Could you check a few things on this model? Use its own coordinates, in mm. Face numbers are marked on the shaded views. A direction names the side the tool comes from. Give positions to 0.01 mm unless a question says otherwise; leave off trailing zeros. Loops run counter-clockwise (first coordinate to the right, second up) from the corner with the lowest first, then second, coordinate; pieces in that order, holes last. Notation, with made-up numbers: M 73.5,-12 L 78.5,-12 A15 cw 78.5,8 Z; hole C -6,-14.75 d7. An arc over 180 degrees is marked long. Answer in a Markdown table with one row per item. Add a question column.
```python
from build123d import *

# Parameters (mm, degrees)
F0_R     = 3
F1_DEPTH = 18.2
F3_DEPTH = 8.5
F5_DEPTH = 14.6
F6_R     = 0.5
F7_DEPTH = 0.5


with BuildPart() as f1:
    # F0 (on Front) → F1 (new body)
    with BuildSketch(Plane.XZ):
        with BuildLine():
            Line((-15.090977, -27.410671), (-15.090977, -30.910671))
            Line((-15.090977, -30.910671), (-3.590977, -30.910671))
            Line((-3.590977, -30.910671), (-3.590977, -27.410671))
            Line((-3.590977, -27.410671), (-2.840977, -27.410671))
            Line((-2.840977, -27.410671), (-2.840977, -24.910671))
            Line((-2.840977, -24.910671), (-3.590977, -24.910671))
            Line((-3.590977, -24.910671), (-4.440977, -24.910671))
            ThreePointArc((-4.440977, -24.910671), (-5.699463, -22.199699), (-8.290977, -20.710671))
            Line((-8.290977, -20.710671), (-8.290977, -21.210671))
            Line((-8.290977, -21.210671), (-10.390977, -21.210671))
            Line((-10.390977, -21.210671), (-10.390977, -20.710671))
            ThreePointArc((-10.390977, -20.710671), (-12.982492, -22.199699), (-14.240977, -24.910671))
            Line((-14.240977, -24.910671), (-15.090977, -24.910671))
            Line((-15.090977, -24.910671), (-15.840977, -24.910671))
            Line((-15.840977, -24.910671), (-15.840977, -27.410671))
            Line((-15.840977, -27.410671), (-15.090977, -27.410671))
        make_face()
        with Locations((-9.340977, -25.910671)):
            Circle(F0_R, mode=Mode.SUBTRACT)
    extrude(amount=F1_DEPTH)

    # F2 (on face) → F3 (join)
    with BuildSketch(Plane.XZ.offset(18.2)):
        with BuildLine():
            Line((-15.090977, -27.410671), (-15.090977, -30.910671))
            Line((-15.090977, -30.910671), (-3.590977, -30.910671))
            Line((-3.590977, -30.910671), (-3.590977, -27.410671))
            Line((-3.590977, -27.410671), (-2.840977, -27.410671))
            Line((-2.840977, -27.410671), (-2.840977, -24.910671))
            Line((-2.840977, -24.910671), (-3.590977, -24.910671))
            Line((-3.590977, -24.910671), (-4.440977, -24.910671))
            ThreePointArc((-4.440977, -24.910671), (-5.699463, -22.199699), (-8.290977, -20.710671))
            Line((-8.290977, -20.710671), (-8.290977, -21.210671))
            Line((-8.290977, -21.210671), (-10.390977, -21.210671))
            Line((-10.390977, -21.210671), (-10.390977, -20.710671))
            ThreePointArc((-10.390977, -20.710671), (-12.982492, -22.199699), (-14.240977, -24.910671))
            Line((-14.240977, -24.910671), (-15.090977, -24.910671))
            Line((-15.090977, -24.910671), (-15.840977, -24.910671))
            Line((-15.840977, -24.910671), (-15.840977, -27.410671))
            Line((-15.840977, -27.410671), (-15.090977, -27.410671))
        make_face()
    extrude(amount=F3_DEPTH)

    # F4 (on face) → F5 (join)
    with BuildSketch(Plane.XZ.offset(26.7)):
        with BuildLine():
            Line((-15.090977, -27.410671), (-15.090977, -30.910671))
            Line((-15.090977, -30.910671), (-3.590977, -30.910671))
            Line((-3.590977, -30.910671), (-3.590977, -27.410671))
            Line((-3.590977, -27.410671), (-2.840977, -27.410671))
            Line((-2.840977, -27.410671), (-2.840977, -24.910671))
            Line((-2.840977, -24.910671), (-3.590977, -24.910671))
            Line((-3.590977, -24.910671), (-4.440977, -24.910671))
            ThreePointArc((-4.440977, -24.910671), (-5.699463, -22.199699), (-8.290977, -20.710671))
            Line((-8.290977, -20.710671), (-8.290977, -21.210671))
            Line((-8.290977, -21.210671), (-10.390977, -21.210671))
            Line((-10.390977, -21.210671), (-10.390977, -20.710671))
            ThreePointArc((-10.390977, -20.710671), (-12.982492, -22.199699), (-14.240977, -24.910671))
            Line((-14.240977, -24.910671), (-15.090977, -24.910671))
            Line((-15.090977, -24.910671), (-15.840977, -24.910671))
            Line((-15.840977, -24.910671), (-15.840977, -27.410671))
            Line((-15.840977, -27.410671), (-15.090977, -27.410671))
        make_face()
        with BuildLine():
            ThreePointArc((-11.577045, -27.910671), (-9.340977, -22.910671), (-7.104909, -27.910671))
            Line((-7.104909, -27.910671), (-5.340977, -27.910671))
            Line((-5.340977, -27.910671), (-5.340977, -28.910671))
            Line((-5.340977, -28.910671), (-8.840977, -28.910671))
            Line((-8.840977, -28.910671), (-8.840977, -30.310671))
            Line((-8.840977, -30.310671), (-9.840977, -30.310671))
            Line((-9.840977, -30.310671), (-9.840977, -28.910671))
            Line((-9.840977, -28.910671), (-13.340977, -28.910671))
            Line((-13.340977, -28.910671), (-13.340977, -27.910671))
            Line((-13.340977, -27.910671), (-11.577045, -27.910671))
        make_face(mode=Mode.SUBTRACT)
    extrude(amount=F5_DEPTH)

    # F6 (on face) → F7 (cut)
    with BuildSketch(Plane(origin=(0, 0, -30.910671), x_dir=(1, 0, 0), z_dir=(0, 0, -1))):
        with Locations((-13.090977, 39.3)):
            Circle(F6_R)
    extrude(amount=-F7_DEPTH, mode=Mode.SUBTRACT)


solid = f1.part
```
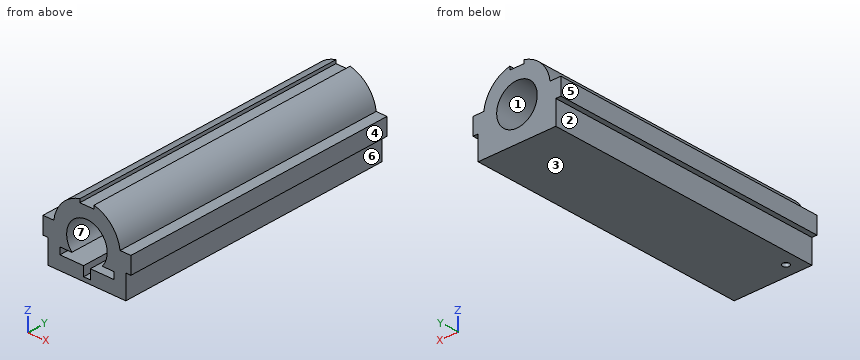
Item 1: Suppose I cut it at C-C (y = -39.3). List the corners of the cut face in (x, z) for me.
Item 2: For P1, Ø0.6, axis at x = -15.5, y = -15.5, coming from the -Z side; P2, Ø1, axis at y = -20, z = -28.5, coming from the -X side; P3, Ø0.6, axis at y = -27, z = -21, coming from the +X side, each with a flat end and sliding along its axis, tell me the tip position at first contact or that it passes through.
Item 3: I need wall thicknesses on L1, parallel to Z at x = -9.5, y = -13; L2, parallel to X at y = -31, z = -30; L3, parallel to Z at x = -9.25, y = -29. Which ranges of each line are inside material? Lowest first, please.
Item 4: For the marked faces 5, 6 and 7, which set-ups out of +Z, -Z, +X, -X, +Y, -Y let a thin tool reach every point of the face, with its end or its side?
Item 5: Suppose I cut it at B-B (z = -29.5). List the corners of the cut face in (x, y) for me, then the cut area to 3 significant figures.
Item 6: Suppose I cut it at A-A (y = -27.5). List the corners of the cut face in (x, z) for me, then the cut area to 3 significant figures.
Item 7: Suppose I cut it at D-D (y = -16). List the corners of the cut face in (x, z) for me.
Item 8: If we mould it in two halves opening along X, with no side actions, what happens to the marked faces 1, 2, 3 and 4? For each: +X half, -X half, draft (parallel to the pull), parting line (faces both ways), or undercut.
Values found:
| question | item | result |
|---|---|---|
| 1 | outline | M -15.84,-27.41 L -15.09,-27.41 L -15.09,-30.91 L -13.59,-30.91 L -13.59,-30.41 L -12.59,-30.41 L -12.59,-30.91 L -3.59,-30.91 L -3.59,-27.41 L -2.84,-27.41 L -2.84,-24.91 L -4.44,-24.91 A4.94 ccw -8.29,-20.71 L -8.29,-21.21 L -10.39,-21.21 L -10.39,-20.71 A4.94 ccw -14.24,-24.91 L -15.84,-24.91 Z; hole M -13.34,-28.91 L -9.84,-28.91 L -9.84,-30.31 L -8.84,-30.31 L -8.84,-28.91 L -5.34,-28.91 L -5.34,-27.91 L -7.1,-27.91 A3 ccw long -11.58,-27.91 L -13.34,-27.91 Z |
| 2 | P1 | z = -27.41 |
| 2 | P2 | x = -15.09 |
| 2 | P3 | x = -6.8 |
| 3 | L1 | -30.91 to -28.91, -22.91 to -21.21 |
| 3 | L2 | -15.09 to -9.84, -8.84 to -3.59 |
| 3 | L3 | -30.91 to -30.31, -22.91 to -21.21 |
| 4 | face 5 | +Z, -Z, -X, +Y, -Y |
| 4 | face 6 | -Z, +X, +Y, -Y |
| 4 | face 7 | -Y |
| 5 | outline | M -15.09,-41.3 L -9.84,-41.3 L -9.84,-26.7 L -8.84,-26.7 L -8.84,-41.3 L -3.59,-41.3 L -3.59,0 L -15.09,0 Z |
| 5 | area | 460 mm² |
| 6 | outline | M -15.84,-27.41 L -15.09,-27.41 L -15.09,-30.91 L -3.59,-30.91 L -3.59,-27.41 L -2.84,-27.41 L -2.84,-24.91 L -4.44,-24.91 A4.94 ccw -8.29,-20.71 L -8.29,-21.21 L -10.39,-21.21 L -10.39,-20.71 A4.94 ccw -14.24,-24.91 L -15.84,-24.91 Z; hole M -13.34,-28.91 L -9.84,-28.91 L -9.84,-30.31 L -8.84,-30.31 L -8.84,-28.91 L -5.34,-28.91 L -5.34,-27.91 L -7.1,-27.91 A3 ccw long -11.58,-27.91 L -13.34,-27.91 Z |
| 6 | area | 69.1 mm² |
| 7 | outline | M -15.84,-27.41 L -15.09,-27.41 L -15.09,-30.91 L -3.59,-30.91 L -3.59,-27.41 L -2.84,-27.41 L -2.84,-24.91 L -4.44,-24.91 A4.94 ccw -8.29,-20.71 L -8.29,-21.21 L -10.39,-21.21 L -10.39,-20.71 A4.94 ccw -14.24,-24.91 L -15.84,-24.91 Z; hole C -9.34,-25.91 d6 |
| 8 | face 1 | undercut |
| 8 | face 2 | -X half |
| 8 | face 3 | draft |
| 8 | face 4 | +X half |
